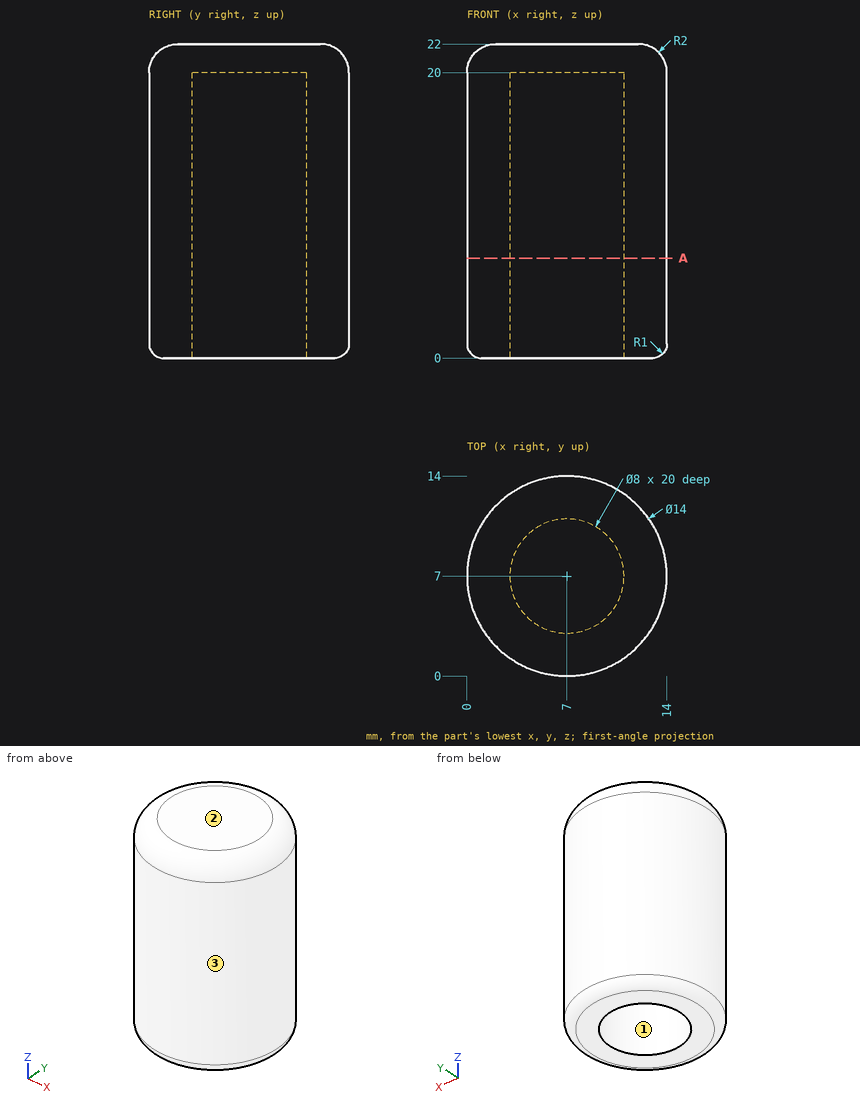
For this review, use the dimensioned drawing (mm, ordinates from the lowest corner) and the shaded views. Coordinates: 2 decimals unless noted, no trailing zeros. Write each loop counter-clockwise with the first axis right and the second up, starting at its lowest first coordinate (ties: lowest second). Pieces come first, ordered by that corner, then holes. Notation, with made-up numbers: (40.5, 76) - (51.5, 76) arc R33 cw to (51.5, 111) - close; hole circle Ø9 at (17, -39). An arc over 180 degrees is marked (long way). One line per item, written item: value.
1) Mouldability with a two-part tool opening along Y and no side actions: class the marked faces 1, 2 and 3 as +Y half, -Y half, draft (parallel to the pull), parting line (faces both ways), or undercut.
Answer sheet:
face 1: undercut
face 2: draft
face 3: parting line
2) To check wall thickness, follow probe 1 along Y at (x, z) = (7, 10.75); probe 2 along Z at (x, y) = (7.5, 10.5); probe 3 along X at (y, z) = (6, 17.75). State the ranges of each line that lie inside material, in increasing order.
Answer sheet:
probe 1: y = 0 to 3, 11 to 14
probe 2: z = 20 to 22
probe 3: x = 0.07 to 3.13, 10.87 to 13.93
3) Insertion check: pin 1 (2 mm diameter, centred on x = 10, z = 16, fed in from -Y); pin 2 (2 mm diameter, centred on y = 12, z = 6.5, fed in from -X); pin 3 (1.5 mm diameter, centred on x = 10, z = 10.5, fed in from +Y). Each pin has a flat end and moves straight along its axis. Give the tip position at first contact, or say it passes through.
Answer sheet:
pin 1: stops at y = 0.29
pin 2: stops at x = 1.26
pin 3: stops at y = 13.63
4) Add section A-A (z = 7). State the section outline as (x, y) points.
Answer sheet:
outline: circle Ø14 at (7, 7); hole circle Ø8 at (7, 7)
